Input: part model. Units: mm. Frame: model coordinates. A direction names the side the tool comes from. Coordinates: 2 decimals unless noted, no trailing zeros. Write each loop counter-clockwise with the first axis right and the second up, starting at its lowest first coordinate (ties: lowest second). Pieces come first, ordered by that corner, then holes. Notation, with made-up numbers: (-25, -27) -> (-5, -27) arc R16 cw to (-5, 2) -> close; hole circle Ø3 at (11.25, 19.5). An arc over 180 degrees is marked (long way). Use one line per item in the form item = value. Start each with the question number.
(1) Ray query, line 1 along Z through (x, y) = (5.85, 27.75); line 2 along X through (y, z) = (25.5, -24.5); line 3 along Z through (x, y) = (1, 5). Return the intervals inside material, ascending.
(2) Set-up query: faces 4 (the face through (16.85, 13.6, 21.14)), 5 (the face through (0.079, 5.07, 26.155)), 6 (the face through (13, 4, -9.5)), 7 (the face through (0, 4, 24.2)), 8 (the face through (0, 20, 20.7)). Return all of +Z, -Z, +X, -X, +Y, -Y with unobstructed straight access to the full face (end or side cutting, diameter ignored); none if empty.
(3) Cut plane D-D on z = -5. Return the cut outline in (x, y).
(4) Pull-direction query (Z, two-part tool) for faces 1 (the face through (0, 0, 26)), 2 (the face through (16.85, 4.31, -7.9)), 3 (the face through (6.12, 24.93, -23.28)); classes: released by +Z, released by -Z, zero draft, split by the parting line, or undercut.
(5) First-contact query: pin 1 (4.5 mm diameter, centred on y = 3.5, z = -23, fed in from +X); pin 2 (1.6 mm diameter, centred on x = -4.5, z = 22.5, fed in from -Y); pin 3 (1.5 mm diameter, centred on x = 5.85, z = -24.5, fed in from +Y); pin 4 (3 mm diameter, centred on x = 14.85, z = 0, fed in from -Y). Flat tips, straight axial feed; report the tip coordinate or a pass-through.
(6) Cut plane A-A on x = -6.75. Return the cut outline in (y, z), plus the area to 3 significant figures.
(7) Cut plane C-C on z = 18.5. Return the cut outline in (x, y), plus the area to 3 significant figures.
(8) Cut plane B-B on y = 18.5. Return the cut outline in (x, z), plus the area to 3 significant figures.
```python
from build123d import *

# Parameters (mm, degrees)
BOSS_EXTRU_1_DEPTH      = 30
ESQUISSE2_W             = 8.5
ESQUISSE2_H             = 19.8
ENL_V_MAT_EXTRU_1_DEPTH = 12
TROU_TARAUD_M31_D       = 2.5
TROU_TARAUD_M31_DEPTH   = 10
TROU_TARAUD_M31_TIP     = 0.751075774
ESQUISSE7_W             = 28
ESQUISSE7_H             = 8.3
BOSS_EXTRU_2_DEPTH      = 18
CHANFREIN3_SIZE         = 3.25
TROU_TARAUD_M32_D       = 2.5
TROU_TARAUD_M32_DEPTH   = 10
TROU_TARAUD_M32_TIP     = 0.751075774
ESQUISSE10_W            = 19.5
ESQUISSE10_H            = 3.5
ENL_V_MAT_EXTRU_2_DEPTH = 10
CHANFREIN4_SIZE         = 1


with BuildPart() as part:
    # Esquisse1 → Boss.-Extru.1 (new body)
    with BuildSketch(Plane(origin=(0, 0, 0), x_dir=(1, 0, 0), z_dir=(0, 1, 0))):
        with BuildLine():
            Line((-9.5, 20.7), (-9.5, 29.3))
            Line((-9.5, 29.3), (18.5, 29.3))
            Line((18.5, 29.3), (18.5, -29.3))
            Line((18.5, -29.3), (-9.5, -29.3))
            Line((-9.5, -29.3), (-9.5, -20.7))
            Line((-9.5, -20.7), (10, -20.7))
            ThreePointArc((10, -20.7), (10.848528137, -20.348528137), (11.2, -19.5))
            Line((11.2, -19.5), (11.2, 19.5))
            ThreePointArc((11.2, 19.5), (10.848528137, 20.348528137), (10, 20.7))
            Line((10, 20.7), (-9.5, 20.7))
        make_face()
    extrude(amount=BOSS_EXTRU_1_DEPTH)

    # Esquisse2 → Enlèv. mat.-Extru.1 (cut)
    with BuildSketch(Plane.XZ):
        with Locations((14.25, 19.4)):
            Rectangle(ESQUISSE2_W, ESQUISSE2_H)
        with Locations((14.25, -19.4)):
            Rectangle(ESQUISSE2_W, ESQUISSE2_H)
    extrude(amount=-ENL_V_MAT_EXTRU_1_DEPTH, mode=Mode.SUBTRACT)

    # Trou taraudé M31
    with Locations(Plane(origin=(0, 0, 0), x_dir=(-1, 0, 0), z_dir=(0, -1, 0))):
        with Locations((-1, 23), (-14.85, 0), (-1, -27)):
            Hole(TROU_TARAUD_M31_D / 2, depth=TROU_TARAUD_M31_DEPTH)
            with Locations((0, 0, -(TROU_TARAUD_M31_DEPTH + TROU_TARAUD_M31_TIP / 2))):  # 118° drill point
                Cone(0, TROU_TARAUD_M31_D / 2, TROU_TARAUD_M31_TIP, mode=Mode.SUBTRACT)

    # Esquisse7 → Boss.-Extru.2 (add)
    with BuildSketch(Plane(origin=(0, 30, 0), x_dir=(1, 0, 0), z_dir=(0, 1, 0))):
        with Locations((4.5, -24.85)):
            Rectangle(ESQUISSE7_W, ESQUISSE7_H)
        with Locations((4.5, 24.85)):
            Rectangle(ESQUISSE7_W, ESQUISSE7_H)
    extrude(amount=-BOSS_EXTRU_2_DEPTH)

    # Chanfrein3
    chanfrein3_edges = [part.edges().sort_by_distance(p)[0] for p in [
        (18.5, 21, -29.3),
        (18.5, 21, 29.3),
        (14.85, 12, 9.5),
        (18.5, 6, 9.5),
        (18.5, 12, 19.4),
        (10, 6, 29.3),
        (10, 6, -29.3),
        (14.85, 12, -9.5),
        (18.5, 12, -19.4),
        (18.5, 6, -9.5),
    ]]
    chamfer(chanfrein3_edges, length=CHANFREIN3_SIZE)

    # Trou taraudé M32
    with Locations(Plane(origin=(0, 30, 0), x_dir=(1, 0, 0), z_dir=(0, 1, 0))):
        with Locations((-4.15, 24.5), (-4.15, -24.5), (5.85, -24.5), (5.85, 24.5)):
            Hole(TROU_TARAUD_M32_D / 2, depth=TROU_TARAUD_M32_DEPTH)
            with Locations((0, 0, -(TROU_TARAUD_M32_DEPTH + TROU_TARAUD_M32_TIP / 2))):  # 118° drill point
                Cone(0, TROU_TARAUD_M32_D / 2, TROU_TARAUD_M32_TIP, mode=Mode.SUBTRACT)

    # Esquisse10 → Enlèv. mat.-Extru.2 (cut)
    with BuildSketch(Plane.XZ):
        with Locations((0.25, 22.45)):
            Rectangle(ESQUISSE10_W, ESQUISSE10_H)
    extrude(amount=-ENL_V_MAT_EXTRU_2_DEPTH, mode=Mode.SUBTRACT)

    # Chanfrein4
    chanfrein4_edges = [part.edges().sort_by_distance(p)[0] for p in [
        (0.25, 10, 24.2),
        (0.25, 10, 20.7),
    ]]
    chamfer(chanfrein4_edges, length=CHANFREIN4_SIZE)


solid = part.part
```
Values:
q1.line_1 = -29.3 to -25.75, -23.25 to -20.7, 20.7 to 23.25, 25.75 to 29.3
q1.line_2 = -9.5 to -5.4, -2.9 to 4.6, 7.1 to 18.5
q1.line_3 = -29.3 to -24.25, -21.75 to -20.7, 24.2 to 25.75, 28.25 to 29.3
q2.face_4 = +Z, +X, -Y
q2.face_5 = -Y
q2.face_6 = -Z, +X, -X, -Y
q2.face_7 = +X, -X, -Y
q2.face_8 = -X, +Y, -Y
q3.outline = (11.2, 0) -> (18.5, 0) -> (18.5, 30) -> (11.2, 30) -> close
q4.face_1 = zero draft
q4.face_2 = released by -Z
q4.face_3 = undercut
q5.pin_1 = 10
q5.pin_2 = 9.9
q5.pin_3 = 19.7
q5.pin_4 = 0
q6.outline = (0, -29.3) -> (30, -29.3) -> (30, -20.7) -> (0, -20.7) -> close; (0, 24.2) -> (9, 24.2) -> (10, 23.2) -> (10, 21.7) -> (11, 20.7) -> (30, 20.7) -> (30, 29.3) -> (0, 29.3) -> close
q6.area = 481 mm2
q7.outline = (11.2, 12) -> (15.25, 12) -> (18.5, 15.25) -> (18.5, 30) -> (11.2, 30) -> close
q7.area = 126 mm2
q8.outline = (-9.5, -29.3) -> (15.25, -29.3) -> (18.5, -26.05) -> (18.5, 26.05) -> (15.25, 29.3) -> (-9.5, 29.3) -> (-9.5, 20.7) -> (10, 20.7) arc R1.2 cw to (11.2, 19.5) -> (11.2, -19.5) arc R1.2 cw to (10, -20.7) -> (-9.5, -20.7) -> close
q8.area = 774 mm2
